Model file for the job. Use its own axes, mm. Round coordinates to 2 decimals unless told otherwise and drop trailing zeros. Order: outer loops, then holes, each group sorted by start corner. A loop starts at its lowest first (then second) coordinate and runs counter-clockwise, first axis right, second up. Notation, with made-up numbers: (-26.5, 2) -> (12.5, 2) arc R12 cw to (12.5, 22) -> close; hole circle Ø4 at (13, 63.5). An arc over 180 degrees is marked (long way). Put each result on its own line as item: value. Start each with the question number.
Q1. Cut at A-A, the plane x = 0. List the corners of the cut face in (y, z), and give its area (3 significant figures).
Q2. Cut at C-C, the plane z = -80. List the corners of the cut face in (x, y).
Q3. Cut at B-B, the plane y = 2.15. List the corners of the cut face in (x, z), and give its area (3 significant figures).
Q4. Probe L1, parallel to X at y = 2.35, z = 0; L2, parallel to X at y = 1.65, z = -80; L3, parallel to Z at x = -3.5, y = 0.45. List the from-to ranges inside material, lowest first.
Q5. Flat gauge pins, fed straight in: P1, Ø1, axis at x = -3.5, z = -76, coming from the -Y side; P2, Ø2, axis at x = -5.5, y = 3.5, coming from the +Z side; P3, Ø2, axis at y = 2.5, z = -76.5, coming from the +X side. Where does each tip first touch, or does it go through?
Q6. Cut at D-D, the plane x = -10.5. List the corners of the cut face in (y, z), and give its area (3 significant figures).
from build123d import *

# Parameters (mm, degrees)
SKETCH1_R           = 18
BOSS_EXTRUDE2_DEPTH = 5.4
SKETCH2_W           = 12
SKETCH2_H           = 90
BOSS_EXTRUDE3_DEPTH = 5.4
SKETCH3_R           = 1.7
SKETCH3_R_2         = 6
CUT_EXTRUDE1_DEPTH  = 92.941068082
CHAMFER1_SIZE       = 4
SKETCH4_R           = 2
CUT_EXTRUDE2_DEPTH  = 92.941068082


with BuildPart() as part:
    # Sketch1 → Boss-Extrude2 (new body)
    with BuildSketch(Plane(origin=(0, 0, 0), x_dir=(1, 0, 0), z_dir=(0, 1, 0))):
        with Locations(Location((0, 0, 0), (0, 0, 90))):
            Circle(SKETCH1_R)
    extrude(amount=BOSS_EXTRUDE2_DEPTH)

    # Sketch2 → Boss-Extrude3 (add)
    with BuildSketch(Plane(origin=(0, 0, 0), x_dir=(1, 0, 0), z_dir=(0, 1, 0))):
        with Locations((0, 45)):
            Rectangle(SKETCH2_W, SKETCH2_H)
    extrude(amount=BOSS_EXTRUDE3_DEPTH)

    # Sketch3 → Cut-Extrude1 (cut, through all)
    with BuildSketch(Plane(origin=(0, 0, 0), x_dir=(1, 0, 0), z_dir=(0, 1, 0))):
        with Locations(Location((10.5, 0, 0), (0, 0, 90))):
            Circle(SKETCH3_R)
        with Locations(Location((0, 0, 0), (0, 0, 90))):
            Circle(SKETCH3_R_2)
        with Locations(Location((0, -10.5, 0), (0, 0, 90))):
            Circle(SKETCH3_R)
        with Locations(Location((-10.5, 0, 0), (0, 0, 90))):
            Circle(SKETCH3_R)
        with Locations(Location((0, 10.5, 0), (0, 0, 90))):
            Circle(SKETCH3_R)
    extrude(amount=CUT_EXTRUDE1_DEPTH, mode=Mode.SUBTRACT)

    # Chamfer1
    chamfer1_edges = [part.edges().sort_by_distance(p)[0] for p in [
        (-6, 2.7, -90),
        (6, 2.7, -90),
    ]]
    chamfer(chamfer1_edges, length=CHAMFER1_SIZE)

    # Sketch4 → Cut-Extrude2 (cut, through all)
    with BuildSketch(Plane(origin=(0, 5.4, 0), x_dir=(1, 0, 0), z_dir=(0, 1, 0))):
        with Locations(Location((0, 80, 0), (0, 0, 270))):
            Circle(SKETCH4_R)
    extrude(amount=-CUT_EXTRUDE2_DEPTH, mode=Mode.SUBTRACT)


solid = part.part
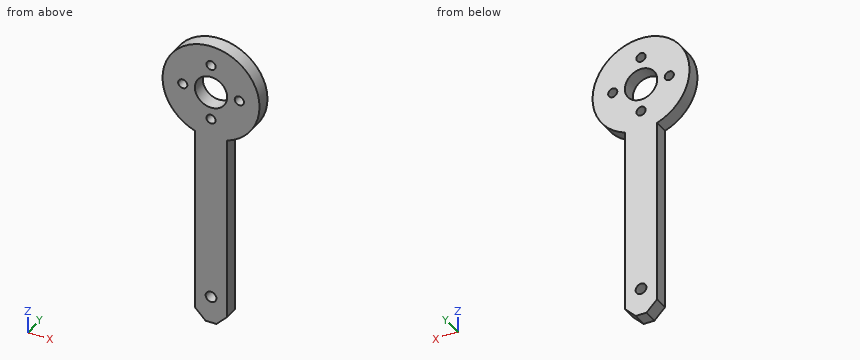
Ans:
1. outline: (0, -90) -> (5.4, -90) -> (5.4, -82) -> (0, -82) -> close; (0, -78) -> (5.4, -78) -> (5.4, -12.2) -> (0, -12.2) -> close; (0, -8.8) -> (5.4, -8.8) -> (5.4, -6) -> (0, -6) -> close; (0, 6) -> (5.4, 6) -> (5.4, 8.8) -> (0, 8.8) -> close; (0, 12.2) -> (5.4, 12.2) -> (5.4, 18) -> (0, 18) -> close
1. area: 460 mm^2
2. outline: (-6, 0) -> (-2, 0) -> (-2, 5.4) -> (-6, 5.4) -> close; (2, 0) -> (6, 0) -> (6, 5.4) -> (2, 5.4) -> close
3. outline: (-6, -86) -> (-2, -90) -> (2, -90) -> (6, -86) -> (6, -16.97) arc R18 ccw (long way) to (-6, -16.97) -> close; hole circle Ø3.4 at (-10.5, 0); hole circle Ø12 at (0, 0); hole circle Ø4 at (0, -80); hole circle Ø3.4 at (0, -10.5); hole circle Ø3.4 at (0, 10.5); hole circle Ø3.4 at (10.5, 0)
3. area: 1,710 mm^2
4. L1: x = -18 to -12.2, -8.8 to -6, 6 to 8.8, 12.2 to 18
4. L2: x = -6 to -2, 2 to 6
4. L3: z = -88.5 to -4.87, 4.87 to 17.66
5. P1: stops at y = 0
5. P2: stops at z = 17.43
5. P3: stops at x = 6
6. outline: (0, -14.62) -> (5.4, -14.62) -> (5.4, -1.7) -> (0, -1.7) -> close; (0, 1.7) -> (5.4, 1.7) -> (5.4, 14.62) -> (0, 14.62) -> close
6. area: 140 mm^2
